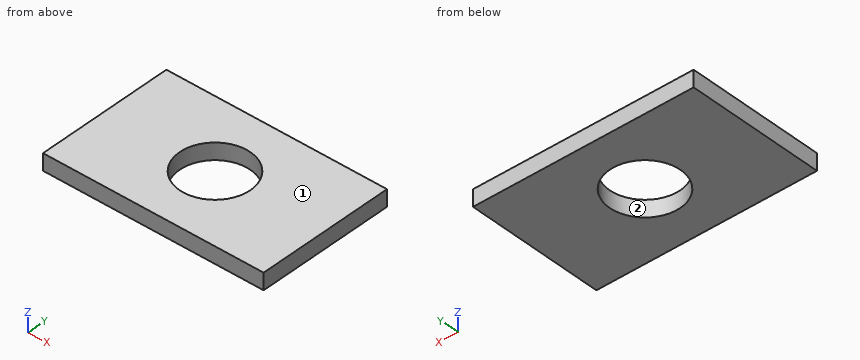
Autodesk Inventor part; units mm, degrees
ref_plane "YZ Plane" through (0, 0, 0) normal (1, 0, 0) x (0, 1, 0)
ref_plane "XZ Plane" through (0, 0, 0) normal (0, 1, 0) x (-1, 0, 0)
ref_plane "XY Plane" through (0, 0, 0) normal (0, 0, 1) x (1, 0, 0)
sketch "Sketch1" plane through (0, 0, 0) normal (0, 0, 1) x (1, 0, 0)
  circle A0 centre (0, 0) radius 6.4
  line L0 (-20, -12.5) -> (20, -12.5)
  line L1 (20, -12.5) -> (20, 12.5)
  line L2 (20, 12.5) -> (-20, 12.5)
  line L3 (-20, 12.5) -> (-20, -12.5)
  dimension "d0" = 12.8
  dimension "d1" = 20
  dimension "d2" = 40
  dimension "d3" = 25
  dimension "d4" = 12.5
extrude "Extrusion1" add sketch "Sketch1" along normal blind 3
properties part number "314-07" material "Steel"
Read the model definition and answer for the solid it produces. Units are mm, in the model's axes. Face numbers are marked on the shaded views. Give positions to 0.01 mm unless a question says otherwise; leave off trailing zeros. Loops run counter-clockwise (first coordinate to the right, second up) from the corner with the lowest first, then second, coordinate; pieces in that order, holes last. Notation, with made-up numbers: (36.5, -23.75) -> (46.5, -23.75) arc R31 ccw to (46.5, 10.25) -> close; hole circle Ø10 at (21, 42.25). An arc over 180 degrees is marked (long way). Use a Markdown table: item, result.
Q1. Determine the mould class of the marked faces 1 and 2 for opening direction X: pulls with the +X half, pulls with the -X half, needs draft (parallel to the pull), parting line crosses it, or undercut.
Solved:
| item | result |
|---|---|
| face 1 | needs draft |
| face 2 | undercut |
Q2. Find the intervals of material crossed by line 1 along Y through (x, z) = (0, 2.6); line 2 along X through (y, z) = (-5.5, 2.35); line 3 along Y through (x, z) = (-1, 0.35), in increasing order.
Solved:
| item | result |
|---|---|
| line 1 | y = -12.5 to -6.4, 6.4 to 12.5 |
| line 2 | x = -20 to -3.27, 3.27 to 20 |
| line 3 | y = -12.5 to -6.32, 6.32 to 12.5 |
Q3. Section C-C, the plane z = 2.1 is taken. Determine the outline of the cut face in (x, y).
Solved:
| item | result |
|---|---|
| outline | (-20, -12.5) -> (20, -12.5) -> (20, 12.5) -> (-20, 12.5) -> close; hole circle Ø12.8 at (0, 0) |
Q4. Section A-A, the plane y = 0 is taken. Determine the outline of the cut face in (x, z).
Solved:
| item | result |
|---|---|
| outline | (-20, 0) -> (-6.4, 0) -> (-6.4, 3) -> (-20, 3) -> close; (6.4, 0) -> (20, 0) -> (20, 3) -> (6.4, 3) -> close |
Q5. Section B-B, the plane x = 0 is taken. Determine the outline of the cut face in (y, z), then the cut area to 3 significant figures.
Solved:
| item | result |
|---|---|
| outline | (-12.5, 0) -> (-6.4, 0) -> (-6.4, 3) -> (-12.5, 3) -> close; (6.4, 0) -> (12.5, 0) -> (12.5, 3) -> (6.4, 3) -> close |
| area | 36.6 mm^2 |
